```python
from build123d import *

# Parameters (mm, degrees)
F0_R     = 2.6
F1_DEPTH = 12.5
F3_DEPTH = 25
F6_DEPTH = 25


with BuildPart() as f1:
    # F0 (on Top) → F1 (new body)
    with BuildSketch(Plane.XY):
        Polygon((3.5, -53), (6.3968370669, -53), (6.3968370669, 53), (3.5, 53), (3.5, 75), (-3.5, 75), (-3.5, 53), (-6.3968370669, 53), (-6.3968370669, -53), (-3.5, -53), (-3.5, -75), (3.5, -75), align=None)
        Circle(F0_R, mode=Mode.SUBTRACT)
    extrude(amount=F1_DEPTH)

    # F2 (on face) → F3 (cut)
    with BuildSketch(Plane.YZ.offset(3.5)):
        with BuildLine():
            Line((69.0972208977, 8.7), (57.500641793, 8.7))
            ThreePointArc((57.500641793, 8.7), (55.050641793, 6.25), (57.500641793, 3.8))
            Line((57.500641793, 3.8), (69.0972208977, 3.8))
            ThreePointArc((69.0972208977, 3.8), (71.5472208977, 6.25), (69.0972208977, 8.7))
        make_face()
    extrude(amount=-F3_DEPTH, mode=Mode.SUBTRACT)

    # F5 (on face) → F6 (cut)
    with BuildSketch(Plane.YZ.offset(3.5)):
        with BuildLine():
            Line((-69.7134453715, 8.7458659336), (-69.6451475877, 8.7458675667))
            ThreePointArc((-69.6451475877, 8.7458675667), (-69.6792964853, 8.7461047508), (-69.7134453715, 8.7458659336))
        make_face()
        with BuildLine():
            Line((-59.7258945025, 8.7461047508), (-69.6451475877, 8.7458675667))
            Line((-69.6451475877, 8.7458675667), (-69.7134453715, 8.7458659336))
            ThreePointArc((-69.7134453715, 8.7458659336), (-72.1291781969, 6.2790006), (-69.6792379022, 3.8461047515))
            Line((-69.6792379022, 3.8461047515), (-59.7258359194, 3.8461047515))
            ThreePointArc((-59.7258359194, 3.8461047515), (-57.2758359196, 6.2961340431), (-59.7258945025, 8.7461047508))
        make_face()
    extrude(amount=-F6_DEPTH, mode=Mode.SUBTRACT)


solid = f1.part
```
Check sheet for the modelled part. Datum: model origin and axes. Units: mm. A direction names the side the tool comes from. Round coordinates to 2 decimals unless told otherwise and drop trailing zeros. Loops run counter-clockwise (first coordinate to the right, second up) from the corner with the lowest first, then second, coordinate; pieces in that order, holes last. Notation, with made-up numbers: (46, 15) - (71, 15) arc R20 cw to (71, 50) - close; hole circle Ø5 at (-33.5, -36). An arc over 180 degrees is marked (long way). Answer as a JSON object with one key per item and string values. Group by question number.
Q1. Sectioned sample at A-A, the plane x = 0. Enter the section's corners in (y, z), plus the area to 3 significant figures.
Q2. Set-up check for faces 1 (the face through (-3.5, 64, 9)), 2 (the face through (3.5, 64, 3)), 3 (the face through (-3.5, -64, 9)), 4 (the face through (3.5, -64, 9)), 5 (the face through (0.049, 71.547, 6.196)): record each of +Z, -Z, +X, -X, +Y, -Y from which the full face is reachable in a straight line by a thin tool's end or side.
Q3. Scan lines: line 1 along Y through (x, z) = (0, 6.5); line 2 along Y through (x, z) = (0, 2.5); line 3 along Y through (x, z) = (0, 7.25). Record each from-to range of solid material in increasing order. Write a range as [from, to].
Q4. Sectioned sample at D-D, the plane y = 0. Enter the section's corners in (x, z).
Q5. Gauge pin test, flat ends, axial feed: P1, Ø6, axis at y = 61, z = 7, coming from the +X side; P2, Ø3, axis at x = 5.5, z = 8.5, coming from the -Y side; P3, Ø2.5, axis at x = -5, z = 8, coming from the +Y side. Record the tip position at first contact, or that the pin passes through.
Q6. Mould release check, pull along Z, two halves, no side actions. Record for faces 6 (the face through (6.397, -1, 6)), 7 (the face through (0, -65, 3.846)), 8 (the face through (0.049, -57.276, 6.242)), 9 (the face through (-3, 1, 0)): released by +Z, released by -Z, zero draft, split by the parting line, or undercut.
Q7. Sectioned sample at C-C, the plane z = 10.25. Enter the section's corners in (x, y), plus the area to 3 significant figures.
Q8. Sectioned sample at B-B, the plane y = 65.5. Enter the section's corners in (x, z), plus the area to 3 significant figures.
Solution:
{
 "1": {"outline": "(-75, 0) - (-2.6, 0) - (-2.6, 12.5) - (-75, 12.5) - close; (2.6, 0) - (75, 0) - (75, 12.5) - (2.6, 12.5) - close; hole (-69.68, 3.85) - (-59.73, 3.85) arc R2.45 ccw to (-59.73, 8.75) - (-69.65, 8.75) arc R2.45 ccw (long way) to start; hole (57.5, 3.8) - (69.1, 3.8) arc R2.45 ccw to (69.1, 8.7) - (57.5, 8.7) arc R2.45 ccw to start", "area": "1,670 mm²"},
 "2": {"face 1": "+Z, -Z, -X, +Y", "face 2": "+Z, -Z, +X, +Y", "face 3": "+Z, -Z, -X, -Y", "face 4": "+Z, -Z, +X, -Y", "face 5": "+X, -X"},
 "3": {"line 1": "y = [-75, -72.12], [-57.28, -2.6], [2.6, 55.06], [71.53, 75]", "line 2": "y = [-75, -2.6], [2.6, 75]", "line 3": "y = [-75, -71.94], [-57.47, -2.6], [2.6, 55.26], [71.33, 75]"},
 "4": {"outline": "(-6.4, 0) - (-2.6, 0) - (-2.6, 12.5) - (-6.4, 12.5) - close; (2.6, 0) - (6.4, 0) - (6.4, 12.5) - (2.6, 12.5) - close"},
 "5": {"P1": "stops at x = 3.5", "P2": "stops at y = -53", "P3": "stops at y = 53"},
 "6": {"face 6": "zero draft", "face 7": "undercut", "face 8": "undercut", "face 9": "released by -Z"},
 "7": {"outline": "(-6.4, -53) - (-3.5, -53) - (-3.5, -75) - (3.5, -75) - (3.5, -53) - (6.4, -53) - (6.4, 53) - (3.5, 53) - (3.5, 75) - (-3.5, 75) - (-3.5, 53) - (-6.4, 53) - close; hole circle Ø5.2 at (0, 0)", "area": "1,640 mm²"},
 "8": {"outline": "(-3.5, 0) - (3.5, 0) - (3.5, 3.8) - (-3.5, 3.8) - close; (-3.5, 8.7) - (3.5, 8.7) - (3.5, 12.5) - (-3.5, 12.5) - close", "area": "53.2 mm²"}
}
